Autodesk Inventor part; units mm, degrees
ref_plane "YZ Plane" through (0, 0, 0) normal (1, 0, 0) x (0, 1, 0)
ref_plane "XZ Plane" through (0, 0, 0) normal (0, 1, 0) x (-1, 0, 0)
ref_plane "XY Plane" through (0, 0, 0) normal (0, 0, 1) x (1, 0, 0)
sketch "Sketch1" plane through (0, 0, 0) normal (0, 1, 0) x (-1, 0, 0)
  circle A0 centre (12.7112, 19.8484) radius 40
  point P0 (0, 0)
extrude "Extrusion1" add sketch "Sketch1" along normal blind 19
sketch "Sketch2" plane through (-12.7112, 19, 19.8484) normal (0, 1, 0) x (1, 0, 0)
  point P0 (12.7112, 19.8484)
sketch "Sketch3" plane through (-12.7112, 19, 19.8484) normal (0, 1, 0) x (1, 0, 0)
  circle A0 centre (0, 0) radius 20
  point P0 (12.7112, 19.8484)
  dimension "d3" = 40
extrude "Extrusion2" add sketch "Sketch3" along normal blind 7
sketch "Sketch4" plane through (-12.7112, 26, 19.8484) normal (0, 1, 0) x (1, 0, 0)
  circle A0 centre (0, 0) radius 10
  point P0 (12.7112, 19.8484)
  dimension "d6" = 20
extrude "Extrusion3" cut sketch "Sketch4" against normal blind 4
Can you work these out from the model? Positions are in its coordinate system, mm. A direction names the side the tool comes from. Round coordinates to 2 decimals unless told otherwise and drop trailing zeros. Write each loop counter-clockwise with the first axis right and the second up, starting at its lowest first coordinate (ties: lowest second). Pieces come first, ordered by that corner, then holes. Notation, with made-up numbers: M 63,8 L 85,8 A15 ccw 85,16 Z; hole C 34,32 d9. An arc over 180 degrees is marked long. Use a Markdown table: item, result.
Item 1: Which directions (+Z, -Z, +X, -X, +Y, -Y) give clear straight access to the entire face, cutting with the end or side of a thin tool? Please do faces 4 (the face through (-13, 22, 20)), 5 (the face through (-12, 0, 20)).
Found:
| item | result |
|---|---|
| face 4 | +Y |
| face 5 | +Z, -Z, +X, -X, -Y |
Item 2: For pin 1 Ø12 at (x, z) = (-20.5, 14) entering from +Y; pin 2 Ø10 at (x, y) = (-18.5, 20) entering from -Z; pin 3 Ø5 at (y, z) = (6, -8) entering from +X; pin 4 Ø1.5 at (x, y) = (-33.5, 11) entering from +Z, each with a flat end and sliding along its axis, tell me the tip position at first contact or that it passes through.
Found:
| item | result |
|---|---|
| pin 1 | stops at y = 26 |
| pin 2 | stops at z = -20.14 |
| pin 3 | stops at x = 18.23 |
| pin 4 | stops at z = 54.47 |
Item 3: I want a section at A-A (z = 5.5). List the corners of the cut face in (x, y) for me, and give its area (3 significant figures).
Found:
| item | result |
|---|---|
| outline | M -50.05,0 L 24.63,0 L 24.63,19 L 1.22,19 L 1.22,26 L -26.64,26 L -26.64,19 L -50.05,19 Z |
| area | 1,610 mm2 |
Item 4: We'd pull the mould along X, two halves only. Please class faces 1 (the face through (-22.7, 24, 19.4)), 2 (the face through (-28.6, 22.5, 7.7)), 3 (the face through (6, 19, 12)): released by +X, released by -X, zero draft, split by the parting line, or undercut.
Found:
| item | result |
|---|---|
| face 1 | undercut |
| face 2 | split by the parting line |
| face 3 | zero draft |
Item 5: I want a section at C-C (z = 38.5). List the corners of the cut face in (x, y) for me, and give its area (3 significant figures).
Found:
| item | result |
|---|---|
| outline | M -48.1,0 L 22.67,0 L 22.67,19 L -5.49,19 L -5.49,26 L -19.93,26 L -19.93,19 L -48.1,19 Z |
| area | 1,450 mm2 |
Item 6: I want a section at D-D (y = 23). List the corners of the cut face in (x, z) for me, and give its area (3 significant figures).
Found:
| item | result |
|---|---|
| outline | C -12.71,19.85 d40; hole C -12.71,19.85 d20 |
| area | 942 mm2 |
Item 7: I want a section at B-B (x = -20). List the corners of the cut face in (y, z) for me, and give its area (3 significant figures).
Found:
| item | result |
|---|---|
| outline | M 0,-19.48 L 19,-19.48 L 19,1.22 L 26,1.22 L 26,13 L 22,13 L 22,26.69 L 26,26.69 L 26,38.47 L 19,38.47 L 19,59.18 L 0,59.18 Z |
| area | 1,700 mm2 |
Item 8: If I drill on line 1 along Y through (x, z) = (9.5, 30); line 2 along Z through (x, y) = (-11, 25); line 3 along X through (y, z) = (23.75, 15), over which ranges is the centre line in solid material (lowest first)? Write a range as [from, to].
Found:
| item | result |
|---|---|
| line 1 | y = [0, 19] |
| line 2 | z = [-0.08, 10], [29.7, 39.78] |
| line 3 | x = [-32.11, -21.46], [-3.97, 6.69] |
